```python
from build123d import *

# Parameters (mm, degrees)
F1_DEPTH = 19.05
F3_DEPTH = 9.525
F4_DEPTH = 9.525


with BuildPart() as f1:
    # F0 (on Front) → F1 (new body)
    with BuildSketch(Plane.XZ):
        with BuildLine():
            ThreePointArc((8.512915, 10.469554), (0, -13.49375), (-8.512915, 10.469554))
            ThreePointArc((-8.512915, 10.469554), (-7.617416, 11.979921), (-7.915642, 13.710294))
            ThreePointArc((-7.915642, 13.710294), (-9.654974, 14.938224), (-11.717777, 14.411033))
            ThreePointArc((-11.717777, 14.411033), (0, -18.57375), (11.717777, 14.411033))
            ThreePointArc((11.717777, 14.411033), (9.654974, 14.938224), (7.915642, 13.710294))
            ThreePointArc((7.915642, 13.710294), (7.617416, 11.979921), (8.512915, 10.469554))
        make_face()
    extrude(amount=F1_DEPTH)

    # F2 (on Right) → F3 (join)
    with BuildSketch(Plane.YZ):
        with BuildLine():
            ThreePointArc((-16.7747, -38.108215), (-9.525, -18.57375), (-2.2753, -38.108215))
            ThreePointArc((-2.2753, -38.108215), (-3.122367, -39.607942), (-2.81793, -41.303236))
            ThreePointArc((-2.81793, -41.303236), (-1.043519, -42.537378), (1.038849, -41.958257))
            ThreePointArc((1.038849, -41.958257), (6.653938, -29.02367), (0, -16.59154))
            ThreePointArc((0, -16.59154), (-9.525, -13.49375), (-19.05, -16.59154))
            ThreePointArc((-19.05, -16.59154), (-25.703938, -29.02367), (-20.088849, -41.958257))
            ThreePointArc((-20.088849, -41.958257), (-18.006481, -42.537378), (-16.23207, -41.303236))
            ThreePointArc((-16.23207, -41.303236), (-15.927633, -39.607942), (-16.7747, -38.108215))
        make_face()
    extrude(amount=F3_DEPTH)

    # F2 (on Right) → F4 (join)
    with BuildSketch(Plane.YZ):
        with BuildLine():
            ThreePointArc((-16.7747, -38.108215), (-9.525, -18.57375), (-2.2753, -38.108215))
            ThreePointArc((-2.2753, -38.108215), (-3.122367, -39.607942), (-2.81793, -41.303236))
            ThreePointArc((-2.81793, -41.303236), (-1.043519, -42.537378), (1.038849, -41.958257))
            ThreePointArc((1.038849, -41.958257), (6.653938, -29.02367), (0, -16.59154))
            ThreePointArc((0, -16.59154), (-9.525, -13.49375), (-19.05, -16.59154))
            ThreePointArc((-19.05, -16.59154), (-25.703938, -29.02367), (-20.088849, -41.958257))
            ThreePointArc((-20.088849, -41.958257), (-18.006481, -42.537378), (-16.23207, -41.303236))
            ThreePointArc((-16.23207, -41.303236), (-15.927633, -39.607942), (-16.7747, -38.108215))
        make_face()
    extrude(amount=-F4_DEPTH)


solid = f1.part
```
Input: part model. Units: mm. Frame: model coordinates. A direction names the side the tool comes from. Give positions to 0.01 mm unless a question says otherwise; leave off trailing zeros. Order: outer loops, then holes, each group sorted by start corner. A loop starts at its lowest first (then second) coordinate and runs counter-clockwise, first axis right, second up.
1. Section C-C on z = -33. Return the cut outline in (x, y) (3 decimals), and give its area (3 significant figures).
Derived:
outline: (-9.525, -25.375) - (9.525, -25.375) - (9.525, -20.132) - (-9.525, -20.132) - close; (-9.525, 1.082) - (9.525, 1.082) - (9.525, 6.325) - (-9.525, 6.325) - close
area: 200 mm2
2. Mould query, pull axis Z, two halves, no side actions, for faces 1 (the cylindrical face through (0.464, -9.392, -13.486)), 2 (the flat face through (9.525, -17, -20)). Classes: released by +Z, released by -Z, zero draft, split by the parting line, or undercut.
Derived:
face 1: undercut
face 2: zero draft
3. Reachability of faces 3 (the cylindrical face through (0.13, -9.9, -18.58)), 4 (the flat face through (4, 0, -14)), 5 (the flat face through (-9.525, -17, -20)), 6 (the flat face through (4, -19.05, -14)) from +Z, -Z, +X, -X, +Y, -Y: full face, straight path, thin tool, end or side. Return the list, or none.
Derived:
face 3: +X, -X
face 4: +Z, +X, -X, +Y
face 5: -Z, -X, +Y, -Y
face 6: +Z, +X, -X, -Y
4. Pin query (flat end, axial travel): pin 1 (8 mm diameter, centred on y = -16.5, z = -32.5, fed in from -X) (3 decimals); pin 2 (8 mm diameter, centred on x = 4.5, z = -13.5, fed in from +Y); pin 3 (1 mm diameter, centred on x = -14.5, y = -14, fed in from -Z); pin 4 (1.5 mm diameter, centred on x = 11.5, z = 4.5, fed in from -Y). Return the tip coordinate at first contact, or that it passes through.
Derived:
pin 1: stops at x = -9.525
pin 2: stops at y = 1.14
pin 3: stops at z = -12.21
pin 4: passes through
5. Material intervals for L1, parallel to X at y = -10, z = 0; L2, parallel to Y at x = 0, z = -27; L3, parallel to X at y = -12.5, z = -6, sorted ascending.
Derived:
L1: x = -18.57 to -13.49, 13.49 to 18.57
L2: y = -25.49 to -20.31, 1.26 to 6.44
L3: x = -17.58 to -12.09, 12.09 to 17.58
6. Section A-A on z = 0. Return the cut outline in (x, y).
Derived:
outline: (-18.57, -19.05) - (-13.49, -19.05) - (-13.49, 0) - (-18.57, 0) - close; (13.49, -19.05) - (18.57, -19.05) - (18.57, 0) - (13.49, 0) - close
7. Section D-D on y = -11. Return the cut outline in (x, z) (1 decimal), and give its area (3 significant figures).
Derived:
outline: (-11.7, 14.4) arc R18.6 ccw to (-9.5, -15.9) - (-9.5, -18.7) - (9.5, -18.7) - (9.5, -15.9) arc R18.6 ccw to (11.7, 14.4) arc R2.5 ccw to (7.9, 13.7) arc R2.5 ccw to (8.5, 10.5) arc R13.5 cw (long way) to (-8.5, 10.5) arc R2.5 ccw to (-7.9, 13.7) arc R2.5 ccw to start
area: 439 mm2
